The model under review builds one solid part; all positions refer to its coordinate system, in mm. Round coordinates to 2 decimals unless told otherwise and drop trailing zeros. Loops run counter-clockwise (first coordinate to the right, second up) from the corner with the lowest first, then second, coordinate; pieces in that order, holes last. Notation, with made-up numbers: M -4,21.25 L 30,21.25 A9 ccw 30,30.25 Z; hole C -38.75,-1.75 d10. An arc over 180 degrees is marked long. Use a Markdown table: item, result. Add a question column.
```python
from build123d import *

# Parameters (mm, degrees)
SKETCH1_R           = 15
BOSS_EXTRUDE1_DEPTH = 3


with BuildPart() as part:
    # Sketch1 → Boss-Extrude1 (new body)
    with BuildSketch(Plane.XY):
        Circle(SKETCH1_R)
        with BuildLine():
            ThreePointArc((8.875, 1.494782593), (8.626766656, 2.564936072), (8.25, 3.596873642))
            Line((8.25, 3.596873642), (8.25, 8.25))
            Line((8.25, 8.25), (3.596873642, 8.25))
            ThreePointArc((3.596873642, 8.25), (0, 9), (-3.596873642, 8.25))
            Line((-3.596873642, 8.25), (-8.25, 8.25))
            Line((-8.25, 8.25), (-8.25, 3.596873642))
            ThreePointArc((-8.25, 3.596873642), (-8.626766656, 2.564936072), (-8.875, 1.494782593))
            ThreePointArc((-8.875, 1.494782593), (-10.25, 0), (-8.875, -1.494782593))
            ThreePointArc((-8.875, -1.494782593), (-8.626766656, -2.564936072), (-8.25, -3.596873642))
            Line((-8.25, -3.596873642), (-8.25, -8.25))
            Line((-8.25, -8.25), (-3.596873642, -8.25))
            ThreePointArc((-3.596873642, -8.25), (0, -9), (3.596873642, -8.25))
            Line((3.596873642, -8.25), (8.25, -8.25))
            Line((8.25, -8.25), (8.25, -3.596873642))
            ThreePointArc((8.25, -3.596873642), (8.626766656, -2.564936072), (8.875, -1.494782593))
            ThreePointArc((8.875, -1.494782593), (10.25, 0), (8.875, 1.494782593))
        make_face(mode=Mode.SUBTRACT)
    extrude(amount=BOSS_EXTRUDE1_DEPTH)


solid = part.part
```
(1) Draft analysis for pull direction Y (two halves, no side actions). For faces 1 (the face through (0, -10, 0)), 2 (the face through (-14.985, 0.66, 1.479)), 3 (the face through (8.63, 2.55, 1.48)), state which applies: released by +Y, released by -Y, zero draft, split by the parting line, or undercut.
(2) Consider section D-D, the plane x = 10.75. Give the boundary of the cut face in (y, z), then the cut area to 3 significant figures.
(3) Consider section A-A, the plane y = 0. Give the boundary of the cut face in (x, z).
(4) Consider section C-C, the plane x = -6.25. Give the boundary of the cut face in (y, z), then the cut area to 3 significant figures.
(5) Insertion check: pin 1 Ø1.5 at (y, z) = (-4.5, 0.5) entering from -X; pin 2 Ø0.9 at (x, z) = (6.5, 1) entering from +Y; pin 3 Ø1.5 at (y, z) = (-5.5, 2) entering from +X; pin 4 Ø3 at (x, y) = (-1.5, 10.5) entering from -Z. Each pin has a flat end and moves straight along its axis. Give the tip position at first contact, or say it passes through.
(6) Consider section B-B, the plane z = 0.75. Give the boundary of the cut face in (x, y) (3 decimals), then the cut area to 3 significant figures.
(7) To check wall thickness, follow probe 1 along Y at (x, z) = (-3.75, 0.45); probe 2 along X at (y, z) = (1.25, 1.9); probe 3 along X at (y, z) = (-6, 0.2). State the ranges of each line that lie inside material, in increasing order.
Found:
| question | item | result |
|---|---|---|
| 1 | face 1 | zero draft |
| 1 | face 2 | split by the parting line |
| 1 | face 3 | undercut |
| 2 | outline | M -10.46,0 L 10.46,0 L 10.46,3 L -10.46,3 Z |
| 2 | area | 62.8 mm^2 |
| 3 | outline | M -15,0 L -10.25,0 L -10.25,3 L -15,3 Z; M 10.25,0 L 15,0 L 15,3 L 10.25,3 Z |
| 4 | outline | M -13.64,0 L -8.25,0 L -8.25,3 L -13.64,3 Z; M 8.25,0 L 13.64,0 L 13.64,3 L 8.25,3 Z |
| 4 | area | 32.3 mm^2 |
| 5 | pin 1 | stops at x = -14.52 |
| 5 | pin 2 | stops at y = 13.73 |
| 5 | pin 3 | stops at x = 14.23 |
| 5 | pin 4 | stops at z = 0 |
| 6 | outline | C 0,0 d30; hole M -8.875,-1.495 A9 ccw -8.25,-3.597 L -8.25,-8.25 L -3.597,-8.25 A9 ccw 3.597,-8.25 L 8.25,-8.25 L 8.25,-3.597 A9 ccw 8.875,-1.495 A1.5 ccw 8.875,1.495 A9 ccw 8.25,3.597 L 8.25,8.25 L 3.597,8.25 A9 ccw -3.597,8.25 L -8.25,8.25 L -8.25,3.597 A9 ccw -8.875,1.495 A1.5 ccw Z |
| 6 | area | 414 mm^2 |
| 7 | probe 1 | y = -14.52 to -8.25, 8.25 to 14.52 |
| 7 | probe 2 | x = -14.95 to -9.58, 9.58 to 14.95 |
| 7 | probe 3 | x = -13.75 to -8.25, 8.25 to 13.75 |
